from build123d import *

# Parameters (mm, degrees)
F0_W    = 15.065
F0_H    = 17.4625
F0_W_2  = 7.21
F0_H_2  = 10.285
F2_R    = 1.5875
F3_SIZE = 0.793


with BuildPart() as f1:
    # F0 (on Front) → F1 (revolve)
    with BuildSketch(Plane.XZ):
        with Locations((14.7425, 16.66875)):
            Rectangle(F0_W, F0_H)
        with Locations((3.605, 16.66875)):
            Rectangle(F0_W_2, F0_H)
        with Locations((3.605, 30.5425)):
            Rectangle(F0_W_2, F0_H_2)
    revolve(axis=Axis((11.1375, 0, 0), (1, 0, 0)))

    # F2
    f2_edges = [f1.edges().sort_by_distance(p)[0] for p in [
        (7.21, 0, -25.4),
    ]]
    fillet(f2_edges, radius=F2_R)

    # F3
    f3_edges = [f1.edges().sort_by_distance(p)[0] for p in [
        (22.275, 0, -25.4),
    ]]
    chamfer(f3_edges, length=F3_SIZE)


solid = f1.part
Design review of the part built by this model. Coordinates are the model's own, in mm. A direction names the side the tool comes from. Round coordinates to 2 decimals unless told otherwise and drop trailing zeros. Loops run counter-clockwise (first coordinate to the right, second up) from the corner with the lowest first, then second, coordinate; pieces in that order, holes last. Notation, with made-up numbers: (-15, -14.75) -> (25, -14.75) arc R19 cw to (25, 4.25) -> close; hole circle Ø7 at (81, 87.25). An arc over 180 degrees is marked (long way). Use one line per item in the form item = value. Start each with the question number.
Q1. Machinability: for faces 4 (the face through (7.21, -27, -5)), 5 (the face through (3.66, 21.71, -28.32)), which of the approach directions +Z, -Z, +X, -X, +Y, -Y give a long, thin tool a straight path to every point of the face, cutting with its end or side? Answer none if there is none.
Q2. Wall thickness on line 1 along Z through (x, y) = (20.75, 0); line 2 along Z through (x, y) = (4.5, 0) (1 decimal): over which ranges is each line inside the solid? List them lowest first. Write a range as [from, to].
Q3. Draft analysis for pull direction Z (two halves, no side actions). For faces 1 (the face through (15.051, 24.796, -5.506)), 2 (the face through (0, -0.5, -8.4)), 3 (the face through (11.29, 7.75, -1.72)), state which applies: +Z half, -Z half, draft (parallel to the pull), parting line (faces both ways), or undercut.
Q4. For pin 1 Ø8 at (x, z) = (9.5, -2) entering from -Y (3 decimals); pin 2 Ø12 at (x, y) = (15, 23.5) entering from -Z; pin 3 Ø4 at (x, y) = (6, 14) entering from -Z; pin 4 Ø18.5 at (y, z) = (0, 0) entering from -X, all flat-tipped, find the tip position at first contact; note any pin that passes through.
Q5. We need section D-D on x = 20.25. Give the boundary of the cut face in (y, z) (1 decimal), then the cut area to 3 significant figures.
Q6. We need section C-C on x = 3. Give the boundary of the cut face in (y, z) (1 decimal).
Q7. We need section A-A on z = 0. Give the boundary of the cut face in (x, y) (1 decimal), then the cut area to 3 significant figures.
Calculated:
q1.face_4 = +X
q1.face_5 = +X, -X
q2.line_1 = [-25.4, -7.94], [7.94, 25.4]
q2.line_2 = [-35.7, -7.9], [7.9, 35.7]
q3.face_1 = parting line
q3.face_2 = draft
q3.face_3 = undercut
q4.pin_1 = -35.685
q4.pin_2 = -18.41
q4.pin_3 = -33.61
q4.pin_4 = 0
q5.outline = circle Ø50.8 at (0, 0); hole circle Ø15.9 at (0, 0)
q5.area = 1,830 mm²
q6.outline = circle Ø71.4 at (0, 0); hole circle Ø15.9 at (0, 0)
q7.outline = (0, -35.7) -> (7.2, -35.7) -> (7.2, -27) arc R1.6 cw to (8.8, -25.4) -> (21.5, -25.4) -> (22.3, -24.6) -> (22.3, -7.9) -> (0, -7.9) -> close; (0, 7.9) -> (22.3, 7.9) -> (22.3, 24.6) -> (21.5, 25.4) -> (8.8, 25.4) arc R1.6 cw to (7.2, 27) -> (7.2, 35.7) -> (0, 35.7) -> close
q7.area = 927 mm²
